```python
from build123d import *
from build123d.topology import SkipClean

# Parameters (mm, degrees)
Y_KSEKLIK_EKSTR_ZYON1_DEPTH = 50


with BuildPart() as part:
    # Çizim1 → Yükseklik-Ekstrüzyon1 (new body)
    # profile 1 of 4: a face of its own
    with SkipClean():  # the faces are left unmerged after this step: merging them gives an invalid solid
        with BuildSketch(Plane.XY):
            with BuildLine():
                ThreePointArc((-20, 16), (-18.828427125, 18.828427125), (-16, 20))
                Line((-16, 20), (-4.8, 20))
                ThreePointArc((-4.8, 20), (-4.092893219, 19.707106781), (-3.8, 19))
                Line((-3.8, 19), (-3.8, 16))
                ThreePointArc((-3.8, 16), (-4.092893219, 15.292893219), (-4.8, 15))
                Line((-4.8, 15), (-6.45, 15))
                ThreePointArc((-6.45, 15), (-6.697487373, 15.102512627), (-6.8, 15.35))
                Line((-6.8, 15.35), (-6.8, 17.424871131))
                ThreePointArc((-6.8, 17.424871131), (-6.920871215, 17.689446262), (-7.2, 17.771281292))
                ThreePointArc((-7.2, 17.771281292), (-8.916601049, 16.833030278), (-9.6, 15))
                Line((-9.6, 15), (-9.6, 14))
                ThreePointArc((-9.6, 14), (-7.696194078, 9.403805922), (-3.1, 7.5))
                Line((-3.1, 7.5), (0, 7.5))
                Line((0, 7.5), (0, 3.25))
                ThreePointArc((0, 3.25), (-2.298097039, 2.298097039), (-3.25, 0))
                Line((-3.25, 0), (-7.5, 0))
                Line((-7.5, 0), (-7.5, 3.1))
                ThreePointArc((-7.5, 3.1), (-9.403805922, 7.696194078), (-14, 9.6))
                Line((-14, 9.6), (-15, 9.6))
                ThreePointArc((-15, 9.6), (-16.833030278, 8.916601049), (-17.771281292, 7.2))
                ThreePointArc((-17.771281292, 7.2), (-17.689446262, 6.920871215), (-17.424871131, 6.8))
                Line((-17.424871131, 6.8), (-15.35, 6.8))
                ThreePointArc((-15.35, 6.8), (-15.102512627, 6.697487373), (-15, 6.45))
                Line((-15, 6.45), (-15, 4.8))
                ThreePointArc((-15, 4.8), (-15.292893219, 4.092893219), (-16, 3.8))
                Line((-16, 3.8), (-19, 3.8))
                ThreePointArc((-19, 3.8), (-19.707106781, 4.092893219), (-20, 4.8))
                Line((-20, 4.8), (-20, 16))
            make_face()
            with BuildLine():
                ThreePointArc((-15.8, 17.8), (-17.214213562, 17.214213562), (-17.8, 15.8))
                Line((-17.8, 15.8), (-17.8, 11.8))
                Line((-17.8, 11.8), (-11.8, 11.8))
                Line((-11.8, 11.8), (-11.8, 17.8))
                Line((-11.8, 17.8), (-15.8, 17.8))
            make_face(mode=Mode.SUBTRACT)
        # profile 2 of 4: a face of its own
        with BuildSketch(Plane.XY):
            with BuildLine():
                Line((16, 3.8), (19, 3.8))
                ThreePointArc((19, 3.8), (19.707106781, 4.092893219), (20, 4.8))
                Line((20, 4.8), (20, 16))
                ThreePointArc((20, 16), (18.828427125, 18.828427125), (16, 20))
                Line((16, 20), (4.8, 20))
                ThreePointArc((4.8, 20), (4.092893219, 19.707106781), (3.8, 19))
                Line((3.8, 19), (3.8, 16))
                ThreePointArc((3.8, 16), (4.092893219, 15.292893219), (4.8, 15))
                Line((4.8, 15), (6.45, 15))
                ThreePointArc((6.45, 15), (6.697487373, 15.102512627), (6.8, 15.35))
                Line((6.8, 15.35), (6.8, 17.424871131))
                ThreePointArc((6.8, 17.424871131), (6.920871215, 17.689446262), (7.2, 17.771281292))
                ThreePointArc((7.2, 17.771281292), (8.916601049, 16.833030278), (9.6, 15))
                Line((9.6, 15), (9.6, 14))
                ThreePointArc((9.6, 14), (7.696194078, 9.403805922), (3.1, 7.5))
                Line((3.1, 7.5), (0, 7.5))
                Line((0, 7.5), (0, 3.25))
                ThreePointArc((0, 3.25), (2.298097039, 2.298097039), (3.25, 0))
                Line((3.25, 0), (7.5, 0))
                Line((7.5, 0), (7.5, 3.1))
                ThreePointArc((7.5, 3.1), (9.403805922, 7.696194078), (14, 9.6))
                Line((14, 9.6), (15, 9.6))
                ThreePointArc((15, 9.6), (16.833030278, 8.916601049), (17.771281292, 7.2))
                ThreePointArc((17.771281292, 7.2), (17.689446262, 6.920871215), (17.424871131, 6.8))
                Line((17.424871131, 6.8), (15.35, 6.8))
                ThreePointArc((15.35, 6.8), (15.102512627, 6.697487373), (15, 6.45))
                Line((15, 6.45), (15, 4.8))
                ThreePointArc((15, 4.8), (15.292893219, 4.092893219), (16, 3.8))
            make_face()
        # profile 3 of 4: a face of its own
        with BuildSketch(Plane.XY):
            with BuildLine():
                Line((3.8, -16), (3.8, -19))
                ThreePointArc((3.8, -19), (4.092893219, -19.707106781), (4.8, -20))
                Line((4.8, -20), (16, -20))
                ThreePointArc((16, -20), (18.828427125, -18.828427125), (20, -16))
                Line((20, -16), (20, -4.8))
                ThreePointArc((20, -4.8), (19.707106781, -4.092893219), (19, -3.8))
                Line((19, -3.8), (16, -3.8))
                ThreePointArc((16, -3.8), (15.292893219, -4.092893219), (15, -4.8))
                Line((15, -4.8), (15, -6.45))
                ThreePointArc((15, -6.45), (15.102512627, -6.697487373), (15.35, -6.8))
                Line((15.35, -6.8), (17.424871131, -6.8))
                ThreePointArc((17.424871131, -6.8), (17.689446262, -6.920871215), (17.771281292, -7.2))
                ThreePointArc((17.771281292, -7.2), (16.833030278, -8.916601049), (15, -9.6))
                Line((15, -9.6), (14, -9.6))
                ThreePointArc((14, -9.6), (9.403805922, -7.696194078), (7.5, -3.1))
                Line((7.5, -3.1), (7.5, 0))
                Line((7.5, 0), (3.25, 0))
                ThreePointArc((3.25, 0), (2.298097039, -2.298097039), (0, -3.25))
                Line((0, -3.25), (0, -7.5))
                Line((0, -7.5), (3.1, -7.5))
                ThreePointArc((3.1, -7.5), (7.696194078, -9.403805922), (9.6, -14))
                Line((9.6, -14), (9.6, -15))
                ThreePointArc((9.6, -15), (8.916601049, -16.833030278), (7.2, -17.771281292))
                ThreePointArc((7.2, -17.771281292), (6.920871215, -17.689446262), (6.8, -17.424871131))
                Line((6.8, -17.424871131), (6.8, -15.35))
                ThreePointArc((6.8, -15.35), (6.697487373, -15.102512627), (6.45, -15))
                Line((6.45, -15), (4.8, -15))
                ThreePointArc((4.8, -15), (4.092893219, -15.292893219), (3.8, -16))
            make_face()
        # profile 4 of 4: a face of its own
        with BuildSketch(Plane.XY):
            with BuildLine():
                Line((-16, -3.8), (-19, -3.8))
                ThreePointArc((-19, -3.8), (-19.707106781, -4.092893219), (-20, -4.8))
                Line((-20, -4.8), (-20, -16))
                ThreePointArc((-20, -16), (-18.828427125, -18.828427125), (-16, -20))
                Line((-16, -20), (-4.8, -20))
                ThreePointArc((-4.8, -20), (-4.092893219, -19.707106781), (-3.8, -19))
                Line((-3.8, -19), (-3.8, -16))
                ThreePointArc((-3.8, -16), (-4.092893219, -15.292893219), (-4.8, -15))
                Line((-4.8, -15), (-6.45, -15))
                ThreePointArc((-6.45, -15), (-6.697487373, -15.102512627), (-6.8, -15.35))
                Line((-6.8, -15.35), (-6.8, -17.424871131))
                ThreePointArc((-6.8, -17.424871131), (-6.920871215, -17.689446262), (-7.2, -17.771281292))
                ThreePointArc((-7.2, -17.771281292), (-8.916601049, -16.833030278), (-9.6, -15))
                Line((-9.6, -15), (-9.6, -14))
                ThreePointArc((-9.6, -14), (-7.696194078, -9.403805922), (-3.1, -7.5))
                Line((-3.1, -7.5), (0, -7.5))
                Line((0, -7.5), (0, -3.25))
                ThreePointArc((0, -3.25), (-2.298097039, -2.298097039), (-3.25, 0))
                Line((-3.25, 0), (-7.5, 0))
                Line((-7.5, 0), (-7.5, -3.1))
                ThreePointArc((-7.5, -3.1), (-9.403805922, -7.696194078), (-14, -9.6))
                Line((-14, -9.6), (-15, -9.6))
                ThreePointArc((-15, -9.6), (-16.833030278, -8.916601049), (-17.771281292, -7.2))
                ThreePointArc((-17.771281292, -7.2), (-17.689446262, -6.920871215), (-17.424871131, -6.8))
                Line((-17.424871131, -6.8), (-15.35, -6.8))
                ThreePointArc((-15.35, -6.8), (-15.102512627, -6.697487373), (-15, -6.45))
                Line((-15, -6.45), (-15, -4.8))
                ThreePointArc((-15, -4.8), (-15.292893219, -4.092893219), (-16, -3.8))
            make_face()
        extrude(amount=-Y_KSEKLIK_EKSTR_ZYON1_DEPTH)


solid = part.part
```
The listing builds one solid part. Answer for the finished solid, in the listing's coordinates (mm). A direction names the side the tool comes from. Coordinates: 2 decimals unless noted, no trailing zeros. Order: outer loops, then holes, each group sorted by start corner. A loop starts at its lowest first (then second) coordinate and runs counter-clockwise, first axis right, second up. Notation, with made-up numbers: M 0,43.25 L 44,43.25 A17 ccw 44,50.25 Z; hole C 41,18 d7. An arc over 180 degrees is marked long. Answer as a JSON object with one key per item and string values. Group by question number.
1. A tool of negligible diameter and unlimited length cuts with its end or side. For faces 1 (the flat face through (-7.5, 0, -25)), 2 (the cylindrical face through (16.812, 8.935, -24.65)), 3 (the flat face through (7.5, 0, -25)), 4 (the cylindrical face through (-18.859, 18.797, -24.65)), 5 (the flat face through (20, -10, -25)), from which of +Z, -Z, +X, -X, +Y, -Y can it reach the whole face along a straight path? Write none if from no direction.
2. Section C-C on x = 11 is taken. Write down the section's boundary in (y, z), then the cut area to 3 significant figures.
3. Section D-D on z = -42.5 is taken. State how many separate pieces and enclosed holes the cut face has, then the cut area to 3 significant figures.
4. Determine the mould class of faces 6 (the flat face through (17, 3.8, -25)), 7 (the cylindrical face through (8.935, -16.812, -24.65)), 8 (the cylindrical face through (-18.859, -18.797, -24.65)) for opening direction X: released by +X, released by -X, zero draft, split by the parting line, or undercut.
5. Section A-A on x = -13 is taken. Write down the section's boundary in (y, z), then the cut area to 3 significant figures.
6. Straight lines are drawn through the part: line 1 (X direction, y = 14.5, z = -39); line 2 (X direction, y = 16, z = -43.5); line 3 (X direction, y = 13, z = -41.5). For each, find the intervals that lie inside material, in ascending order.
7. Section B-B on y = -2 is taken. Write down the section's boundary in (x, z).
8. Flat-ended cylindrical pins translate along their axes: P1, Ø1.9, axis at y = 0.5, z = -29, coming from the +X side; P2, Ø5, axis at x = -1.5, z = -18, coming from the -Y side. Find the tip coordinate at first contact, or state that the pin passes through.
Values follow:
{
 "1": {"face 1": "+Z, -Z, -X", "face 2": "+Z, -Z", "face 3": "+Z, -Z, +X", "face 4": "+Z, -Z, -X, +Y", "face 5": "+Z, -Z, +X, +Y, -Y"},
 "2": {"outline": "M -20,-50 L -8.87,-50 L -8.87,0 L -20,0 Z; M 8.87,-50 L 20,-50 L 20,0 L 8.87,0 Z", "area": "1,110 mm2"},
 "3": {"separate pieces": "1", "enclosed holes": "2", "area": "810 mm2"},
 "4": {"face 6": "zero draft", "face 7": "undercut", "face 8": "released by -X"},
 "5": {"outline": "M -20,-50 L -9.52,-50 L -9.52,0 L -20,0 Z; M 9.52,-50 L 11.8,-50 L 11.8,0 L 9.52,0 Z; M 17.8,-50 L 20,-50 L 20,0 L 17.8,0 Z", "area": "748 mm2"},
 "6": {"line 1": "-20 to -17.8, -11.8 to -9.6, 9.6 to 20", "line 2": "-20 to -17.79, -11.8 to -9.42, -6.8 to -3.8, 3.8 to 6.8, 9.42 to 20", "line 3": "-20 to -17.8, -11.8 to -9.52, 9.52 to 20"},
 "7": {"outline": "M -7.5,-50 L -2.56,-50 L -2.56,0 L -7.5,0 Z; M 2.56,-50 L 7.5,-50 L 7.5,0 L 2.56,0 Z"},
 "8": {"P1": "x = 7.5", "P2": "y = -19.6"}
}
